Source: CAD feature listing. Evaluate the final solid. Frame: model axes, mm. Round coordinates to 2 decimals unless told otherwise and drop trailing zeros. Order: outer loops, then holes, each group sorted by start corner. A loop starts at its lowest first (then second) coordinate and runs counter-clockwise, first axis right, second up. Notation, with made-up numbers: M -16,-28.5 L 13,-28.5 A26 ccw 13,10.5 Z; hole C 40,7 d4. An arc over 180 degrees is marked long. Use one line per item in the form item = value. Start each with the question number.
Q1. Contact query for flat-ended pins moving along their axis: pin 1 (2.5 mm diameter, centred on x = 7.5, z = 10.5, fed in from +Y); pin 2 (4 mm diameter, centred on y = -25, z = 84, fed in from -X). Output: stop coordinate, or through.
Q2. Section A-A (z = 142). Return the cut outline in (x, y).
Q3. Pull-direction query (Y, two-part tool) for faces 1 (the flat face through (5, -100, 2)), 2 (the flat face through (5, -39, -162)), 3 (the cylindrical face through (5, -10, -3)); classes: pulls with the +Y half, pulls with the -Y half, needs draft (parallel to the pull), parting line crosses it, or undercut.
Q4. Material intervals for probe 1 along Y at (x, z) = (5, -153); probe 2 along Y at (x, z) = (4.25, -25); probe 3 along Y at (x, z) = (5, -10), sorted ascending.
Q5. Section B-B (y = -3.5). Return the cut outline in (x, z), plus the area to 3 significant figures.
Q6. Section C-C (z = 99.5). Return the cut outline in (x, y), plus the area to 3 significant figures.
from build123d import *

# Parameters (mm, degrees)
SKETCH1_W                                            = 324
SKETCH1_H                                            = 40
BOSS_EXTRUDE1_DEPTH                                  = 10
G1_4_TAPPED_HOLE1_D                                  = 6
CSK_FOR_M3_COUNTERSUNK_FLAT_HEAD1_D                  = 3.4
CSK_FOR_M3_COUNTERSUNK_FLAT_HEAD1_CSINK_D            = 6.3
CSK_FOR_M3_COUNTERSUNK_FLAT_HEAD1_CSINK_ANGLE        = 90
SKETCH9_W                                            = 10
SKETCH9_H                                            = 324
BOSS_EXTRUDE2_DEPTH                                  = 80
CSK_FOR_M3_COUNTERSUNK_FLAT_HEAD2_D                  = 3.4
CSK_FOR_M3_COUNTERSUNK_FLAT_HEAD2_DEPTH              = 11.5
CSK_FOR_M3_COUNTERSUNK_FLAT_HEAD2_CSINK_D            = 6.3
CSK_FOR_M3_COUNTERSUNK_FLAT_HEAD2_CSINK_ANGLE        = 90
CSK_FOR_M3_COUNTERSUNK_FLAT_HEAD2_TIP                = 1.021463052
M3X0_5_TAPPED_HOLE1_AT_2_COUNT                       = 2
M3X0_5_TAPPED_HOLE1_AT_2_PITCH                       = 25
M3X0_5_TAPPED_HOLE1_AT_3_COUNT                       = 2
M3X0_5_TAPPED_HOLE1_AT_3_PITCH                       = 50
M3X0_5_TAPPED_HOLE1_AT_4_COUNT                       = 2
M3X0_5_TAPPED_HOLE1_AT_4_PITCH                       = 75
SKETCH14_W                                           = 8
SKETCH14_H                                           = 324
CUT_EXTRUDE1_DEPTH                                   = 1
CSK_FOR_M3_CROSS_RECESS_FLAT_HEAD_SCREW1_D           = 3.4
CSK_FOR_M3_CROSS_RECESS_FLAT_HEAD_SCREW1_CSINK_D     = 6.3
CSK_FOR_M3_CROSS_RECESS_FLAT_HEAD_SCREW1_CSINK_ANGLE = 90
LPATTERN1_COUNT                                      = 4
LPATTERN1_PITCH                                      = 42
LPATTERN1_COL_COUNT                                  = 4
LPATTERN1_COL_PITCH                                  = 42
M20X1_5_TAPPED_HOLE1_D                               = 18.5


with BuildPart() as part:
    # Sketch1 → Boss-Extrude1 (new body)
    with BuildSketch(Plane(origin=(0, 0, 0), x_dir=(0, 0, -1), z_dir=(1, 0, 0))):
        Rectangle(SKETCH1_W, SKETCH1_H)
    extrude(amount=BOSS_EXTRUDE1_DEPTH)

    # G1/4 Tapped Hole1 (through all)
    with Locations(Plane(origin=(0, -10, 0), x_dir=(0, 0, -1), z_dir=(-1, 0, 0))):
        with Locations((0, 0)):
            Hole(G1_4_TAPPED_HOLE1_D / 2)

    # CSK for M3 Countersunk Flat Head1 (through all)
    with Locations(Plane(origin=(0, -10, -10), x_dir=(0, 0, -1), z_dir=(-1, 0, 0))):
        with Locations((0, 0)):
            csk_for_m3_countersunk_flat_head1 = CounterSinkHole(CSK_FOR_M3_COUNTERSUNK_FLAT_HEAD1_D / 2, CSK_FOR_M3_COUNTERSUNK_FLAT_HEAD1_CSINK_D / 2, counter_sink_angle=CSK_FOR_M3_COUNTERSUNK_FLAT_HEAD1_CSINK_ANGLE)

    # Mirror1: CSK for M3 Countersunk Flat Head1 across plane
    add(csk_for_m3_countersunk_flat_head1.mirror(Plane.XY), mode=Mode.SUBTRACT)

    # Sketch9 → Boss-Extrude2 (add)
    with BuildSketch(Plane.XZ.offset(20)):
        with Locations((5, 0)):
            Rectangle(SKETCH9_W, SKETCH9_H)
    extrude(amount=BOSS_EXTRUDE2_DEPTH)

    # CSK for M3 Countersunk Flat Head2
    with Locations(Plane(origin=(10, -96, 125), x_dir=(0, 0, 1), z_dir=(1, 0, 0))):
        with Locations((0, 0), (-50, 0), (-100, 0), (-150, 0), (-200, 0), (-250, 0)):
            CounterSinkHole(CSK_FOR_M3_COUNTERSUNK_FLAT_HEAD2_D / 2, CSK_FOR_M3_COUNTERSUNK_FLAT_HEAD2_CSINK_D / 2, depth=CSK_FOR_M3_COUNTERSUNK_FLAT_HEAD2_DEPTH, counter_sink_angle=CSK_FOR_M3_COUNTERSUNK_FLAT_HEAD2_CSINK_ANGLE)
            with Locations((0, 0, -(CSK_FOR_M3_COUNTERSUNK_FLAT_HEAD2_DEPTH + CSK_FOR_M3_COUNTERSUNK_FLAT_HEAD2_TIP / 2))):  # 118° drill point
                Cone(0, CSK_FOR_M3_COUNTERSUNK_FLAT_HEAD2_D / 2, CSK_FOR_M3_COUNTERSUNK_FLAT_HEAD2_TIP, mode=Mode.SUBTRACT)

    # Sketch13 → M3x0.5 Tapped Hole1 (revolve, cut)
    with BuildSketch(Plane(origin=(5, 7.5, 162), x_dir=(0, -1, 0), z_dir=(1, 0, 0))):
        Polygon((0, 0), (0, 12.251075774), (1.25, 11.5), (1.25, 0), align=None)
    m3x0_5_tapped_hole1 = revolve(axis=Axis((5, 7.5, 168.35), (0, 0, -1)), mode=Mode.SUBTRACT)

    # M3x0.5 Tapped Hole1 at 2: M3x0.5 Tapped Hole1 ×2
    with Locations(*[(0, -i * M3X0_5_TAPPED_HOLE1_AT_2_PITCH, 0) for i in range(1, M3X0_5_TAPPED_HOLE1_AT_2_COUNT)]):
        add(m3x0_5_tapped_hole1, mode=Mode.SUBTRACT)

    # M3x0.5 Tapped Hole1 at 3: M3x0.5 Tapped Hole1 ×2
    with Locations(*[(0, -i * M3X0_5_TAPPED_HOLE1_AT_3_PITCH, 0) for i in range(1, M3X0_5_TAPPED_HOLE1_AT_3_COUNT)]):
        add(m3x0_5_tapped_hole1, mode=Mode.SUBTRACT)

    # M3x0.5 Tapped Hole1 at 4: M3x0.5 Tapped Hole1 ×2
    with Locations(*[(0, -i * M3X0_5_TAPPED_HOLE1_AT_4_PITCH, 0) for i in range(1, M3X0_5_TAPPED_HOLE1_AT_4_COUNT)]):
        add(m3x0_5_tapped_hole1, mode=Mode.SUBTRACT)

    # Mirror2: M3x0.5 Tapped Hole1 across plane
    add(m3x0_5_tapped_hole1.mirror(Plane.XY), mode=Mode.SUBTRACT)

    # Mirror2 copy 1 sketch → Mirror2 copy 1 (revolve, cut)
    with BuildSketch(Plane(origin=(5, -17.5, -162), x_dir=(0, -1, 0), z_dir=(1, 0, 0))):
        Polygon((0, 0), (0, -12.251075774), (1.25, -11.5), (1.25, 0), align=None)
    revolve(axis=Axis((5, -17.5, -168.35), (0, 0, -1)), mode=Mode.SUBTRACT)

    # Mirror2 copy 2 sketch → Mirror2 copy 2 (revolve, cut)
    with BuildSketch(Plane(origin=(5, -42.5, -162), x_dir=(0, -1, 0), z_dir=(1, 0, 0))):
        Polygon((0, 0), (0, -12.251075774), (1.25, -11.5), (1.25, 0), align=None)
    revolve(axis=Axis((5, -42.5, -168.35), (0, 0, -1)), mode=Mode.SUBTRACT)

    # Mirror2 copy 3 sketch → Mirror2 copy 3 (revolve, cut)
    with BuildSketch(Plane(origin=(5, -67.5, -162), x_dir=(0, -1, 0), z_dir=(1, 0, 0))):
        Polygon((0, 0), (0, -12.251075774), (1.25, -11.5), (1.25, 0), align=None)
    revolve(axis=Axis((5, -67.5, -168.35), (0, 0, -1)), mode=Mode.SUBTRACT)

    # Sketch14 → Cut-Extrude1 (cut)
    with BuildSketch(Plane(origin=(0, 20, 0), x_dir=(1, 0, 0), z_dir=(0, 1, 0))):
        with Locations((6, 0)):
            Rectangle(SKETCH14_W, SKETCH14_H)
    extrude(amount=-CUT_EXTRUDE1_DEPTH, mode=Mode.SUBTRACT)

    # CSK for M3 Cross Recess Flat Head Screw1 (through all)
    with Locations(Plane(origin=(0, -25, 0), x_dir=(0, 0, -1), z_dir=(-1, 0, 0))):
        with Locations((0, 0)):
            csk_for_m3_cross_recess_flat_head_screw1 = CounterSinkHole(CSK_FOR_M3_CROSS_RECESS_FLAT_HEAD_SCREW1_D / 2, CSK_FOR_M3_CROSS_RECESS_FLAT_HEAD_SCREW1_CSINK_D / 2, counter_sink_angle=CSK_FOR_M3_CROSS_RECESS_FLAT_HEAD_SCREW1_CSINK_ANGLE)

    # LPattern1: CSK for M3 Cross Recess Flat Head Screw1 ×4
    with Locations(*[(0, 0, i * LPATTERN1_PITCH) for i in range(1, LPATTERN1_COUNT)]):
        add(csk_for_m3_cross_recess_flat_head_screw1, mode=Mode.SUBTRACT)

    # LPattern1 col: CSK for M3 Cross Recess Flat Head Screw1 ×4
    with Locations(*[(0, 0, -i * LPATTERN1_COL_PITCH) for i in range(1, LPATTERN1_COL_COUNT)]):
        add(csk_for_m3_cross_recess_flat_head_screw1, mode=Mode.SUBTRACT)

    # M20x1.5 Tapped Hole1 (through all)
    with Locations(Plane(origin=(0, -9, 142), x_dir=(0, 0, -1), z_dir=(-1, 0, 0))):
        with Locations((0, 0), (284, 0), (40, 0)):
            Hole(M20X1_5_TAPPED_HOLE1_D / 2)


solid = part.part
Results list:
q1.pin_1 = 19
q1.pin_2 = 1.15
q2.outline = M 0,-100 L 10,-100 L 10,-18.25 L 0,-18.25 Z; M 0,0.25 L 10,0.25 L 10,19 L 2,19 L 2,20 L 0,20 Z
q3.face_1 = pulls with the -Y half
q3.face_2 = needs draft
q3.face_3 = undercut
q4.probe_1 = -100 to -68.75, -66.25 to -43.75, -41.25 to -18.75, -16.25 to 6.25, 8.75 to 19
q4.probe_2 = -100 to -97.7, -94.3 to 19
q4.probe_3 = -100 to -11.7, -8.3 to 19
q5.outline = M 0,-162 L 10,-162 L 10,-149.44 L 0,-149.44 Z; M 0,-134.56 L 10,-134.56 L 10,94.56 L 0,94.56 Z; M 0,109.44 L 10,109.44 L 10,134.56 L 0,134.56 Z; M 0,149.44 L 10,149.44 L 10,162 L 0,162 Z
q5.area = 2,790 mm2
q6.outline = M 0,-100 L 10,-100 L 10,-17.91 L 0,-17.91 Z; M 0,-0.09 L 10,-0.09 L 10,19 L 2,19 L 2,20 L 0,20 Z
q6.area = 1,010 mm2
